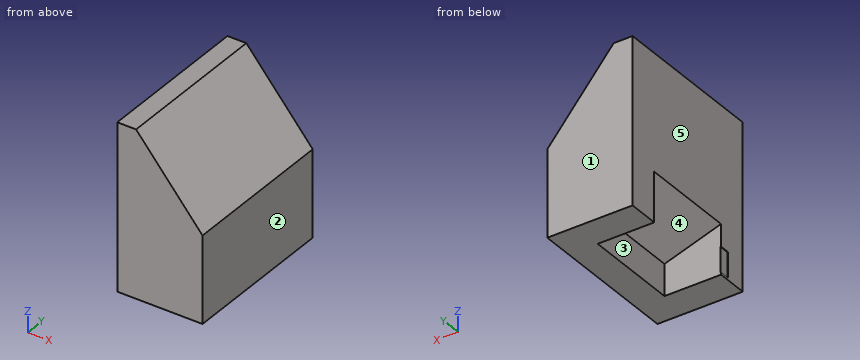
from build123d import *

# Parameters (mm, degrees)
SKETCH1_W           = 37.7
SKETCH1_H           = 80.8
BOSS_EXTRUDE1_DEPTH = 35
CAVITY1_START       = -21.21
CAVITY1_DEPTH       = 42.42
CAVITY1_START_2     = -25.755
CAVITY1_2_OUTLINE_W = 0.255
CAVITY1_2_OUTLINE_H = 11.11
CAVITY1_2_DEPTH     = 4.545
CUT_EXTRUDE1_DEPTH  = 91.031327881
CUT_EXTRUDE2_DEPTH  = 7.5


# Read off the part's stored shape, not the designer's step: Cavity1
with BuildPart() as part:
    # Sketch1 → Boss-Extrude1 (new, symmetric)
    with BuildSketch(Plane(origin=(0, 0, 0), x_dir=(1, 0, 0), z_dir=(0, 1, 0))):
        with Locations((-6.15, -10.4)):
            Rectangle(SKETCH1_W, SKETCH1_H)
    extrude(amount=BOSS_EXTRUDE1_DEPTH, both=True)

    # Cavity1 outline → Cavity1 (cut)
    with BuildSketch(Plane(origin=(0, 0, 0), x_dir=(1, 0, 0), z_dir=(0, 1, 0)).offset(CAVITY1_START)):
        Polygon((0, 8.585), (0, 30), (-25, 30), (-25, 0.566132075), align=None)
    extrude(amount=CAVITY1_DEPTH, mode=Mode.SUBTRACT)

    # Cavity1 2 outline → Cavity1 2 (cut)
    with BuildSketch(Plane(origin=(0, 0, 0), x_dir=(1, 0, 0), z_dir=(0, 1, 0)).offset(CAVITY1_START_2)):
        with Locations((-24.8725, 15.9075)):
            Rectangle(CAVITY1_2_OUTLINE_W, CAVITY1_2_OUTLINE_H)
    extrude(amount=CAVITY1_2_DEPTH, mode=Mode.SUBTRACT)

    # Sketch2 → Cut-Extrude1 (cut, through all)
    with BuildSketch(Plane(origin=(0, 35, 0), x_dir=(1, 0, 0), z_dir=(0, 1, 0))):
        Polygon((12.7, -15.795114576), (-16.672586448, -50.8), (12.7, -50.8), align=None)
    extrude(amount=-CUT_EXTRUDE1_DEPTH, mode=Mode.SUBTRACT)

    # Sketch3 → Cut-Extrude2 (cut)
    with BuildSketch(Plane(origin=(0, 0, -30), x_dir=(-1, 0, 0), z_dir=(0, 0, -1))):
        Polygon((-12.7, 35), (25, 35), (25, 21.21), (0, 21.21), (0, -21.21), (25, -21.21), (25, -35), (-12.7, -35), align=None)
    extrude(amount=-CUT_EXTRUDE2_DEPTH, mode=Mode.SUBTRACT)


solid = part.part
Could you check a few things on this model? Use its own coordinates, in mm. Face numbers are marked on the shaded views. A direction names the side the tool comes from. Give positions to 0.01 mm unless a question says otherwise; leave off trailing zeros. Order: outer loops, then holes, each group sorted by start corner. A loop starts at its lowest first (then second) coordinate and runs counter-clockwise, first axis right, second up. Notation, with made-up numbers: (2.25, 11) - (44.25, 11) arc R20 ccw to (44.25, 36) - close; hole circle Ø9 at (-35.75, -16). An arc over 180 degrees is marked (long way). One line per question, with ' | ' between items. Start each with the question number.
Item 1: I'm going to push flat-ended pins straight in: pin 1 Ø1.4 at (y, z) = (-24, -18) entering from -X (3 decimals); pin 2 Ø4 at (x, y) = (-2, 13.5) entering from +Z; pin 3 Ø4 at (y, z) = (2.5, 20.5) entering from +X. Where does each tip first touch, or does it pass through?
Item 2: For the marked faces 4 and 5, which set-ups out of +Z, -Z, +X, -X, +Y, -Y let a thin tool reach every point of the face, with its end or its side?
Item 3: I want a section at B-B on z = -16. Write out the boundary of the cut face in (x, y) (3 decimals), then the cut area to 3 significant figures.
Item 4: I want a section at C-C on x = -2.5. Write out the boundary of the cut face in (y, z), then the cut area to 3 significant figures.
Item 5: I want a section at A-A on y = 18. Write out the boundary of the cut face in (x, z) (3 decimals), then the cut area to 3 significant figures.
Item 6: I want a section at D-D on y = -30.5. Write out the boundary of the cut face in (x, z), then the cut area to 3 significant figures.
Item 7: I need wall thicknesses on probe 1 along Y at (x, z) = (-20, -4); probe 2 along Z at (x, y) = (3.5, -29); probe 3 along X at (y, z) = (19, 24). Which ranges of each line are inside material? Lowest first, please. Write a range as [from, to].
Item 8: Thinking about a two-plate mould opening in Y: for the marked faces 1, 2 and 3, which applies, pulls with the +Y half, pulls with the -Y half, needs draft (parallel to the pull), parting line crosses it, or undercut?
Verdict:
1) pin 1: x = -24.745 | pin 2: z = 35.7 | pin 3: x = 10.43
2) face 4: -Z, -X | face 5: +Z, -Z, -X, +Y, -Y
3) outline: (-25, -35) - (12.7, -35) - (12.7, 35) - (-25, 35) - (-25, 21.21) - (0, 21.21) - (0, -21.21) - (-24.745, -21.21) - (-24.745, -25.755) - (-25, -25.755) - close | area: 1,580 mm^2
4) outline: (-35, -22.5) - (-21.21, -22.5) - (-21.21, -7.78) - (21.21, -7.78) - (21.21, -22.5) - (35, -22.5) - (35, 33.91) - (-35, 33.91) - close | area: 3,320 mm^2
5) outline: (-25, -0.566) - (0, -8.585) - (0, -22.5) - (12.7, -22.5) - (12.7, 15.795) - (-16.673, 50.8) - (-25, 50.8) - close | area: 1,800 mm^2
6) outline: (-25, -22.5) - (12.7, -22.5) - (12.7, 15.8) - (-16.67, 50.8) - (-25, 50.8) - close | area: 2,250 mm^2
7) probe 1: [-35, -21.21], [21.21, 35] | probe 2: [-22.5, 26.76] | probe 3: [-25, 5.82]
8) face 1: pulls with the +Y half | face 2: needs draft | face 3: undercut
